```python
from build123d import *

# Parameters (mm, degrees)
SKETCH1_W               = 5.7
SKETCH1_H               = 3.4
SKETCH1_W_2             = 36.24
SKETCH1_H_2             = 45
BOSS_EXTRUDE1_DEPTH     = 3
CUT_EXTRUDE1_DEPTH      = 61
CUT_EXTRUDE1_DEPTH_BACK = 19
SKETCH3_W               = 24.5
SKETCH3_H               = 2.46523088
BOSS_EXTRUDE2_DEPTH     = 2


with BuildPart() as part:
    # Sketch1 → Boss-Extrude1 (new body)
    with BuildSketch(Plane(origin=(0, 0, 0), x_dir=(1, 0, 0), z_dir=(0, 1, 0))):
        Polygon((85, 0), (0, 0), (0, -23), (8.59, -23), (8.59, -32), (0, -32), (0, -55), (85, -55), align=None)
        Polygon((9.59, -33.35), (9.59, -32.35), (9.59, -22.65), (9.59, -21.65), (13.68, -21.65), (13.68, -33.35), align=None, mode=Mode.SUBTRACT)
        with Locations((73.3, -27.5)):
            Rectangle(SKETCH1_W, SKETCH1_H, mode=Mode.SUBTRACT)
        with Locations((45.38, -27.5)):
            Rectangle(SKETCH1_W_2, SKETCH1_H_2, mode=Mode.SUBTRACT)
    extrude(amount=BOSS_EXTRUDE1_DEPTH)

    # Sketch3 → Cut-Extrude1 (cut, two sides: drawn at the far end of the back side and taken through both)
    with BuildSketch(Plane.ZY.offset(-63.5).offset(-CUT_EXTRUDE1_DEPTH_BACK)):
        with Locations((27.5, 1.23261544)):
            Rectangle(SKETCH3_W, SKETCH3_H)
    extrude(amount=CUT_EXTRUDE1_DEPTH + CUT_EXTRUDE1_DEPTH_BACK, mode=Mode.SUBTRACT)

    # Sketch4 → Boss-Extrude2 (add)
    with BuildSketch(Plane.XZ):
        Polygon((0, 32), (2.5, 32), (2.5, 39.75), (2.5, 52.5), (82.5, 52.5), (82.5, 39.75), (82.5, 15.25), (82.5, 2.5), (2.5, 2.5), (2.5, 15.25), (2.5, 23), (0, 23), (0, 0), (85, 0), (85, 55), (0, 55), align=None)
    extrude(amount=BOSS_EXTRUDE2_DEPTH)


solid = part.part
```
Geometry: final body of the model. Coordinates: model frame, mm. A direction names the side the tool comes from. Give positions to 0.01 mm unless a question says otherwise; leave off trailing zeros. Write each loop counter-clockwise with the first axis right and the second up, starting at its lowest first coordinate (ties: lowest second). Pieces come first, ordered by that corner, then holes.
1. Section query C-C, the plane y = 0.8. Return loops of the section in (x, z), then the cut area to 3 significant figures.
2. Draft query along X for faces 1 (the flat face through (0, 1, 44)), 2 (the flat face through (43, 1, 55)), 3 (the flat face through (42, -1, 52.5)). Return one class per face: released by +X, released by -X, zero draft, split by the parting line, or undercut.
3. Section query D-D, the plane x = 57. Return loops of the section in (y, z).
4. Section query B-B, the plane x = 19. Return loops of the section in (y, z).
5. Reachability of faces 4 (the flat face through (27.26, 2.8, 27.8)), 5 (the flat face through (2, 1, 32)), 6 (the flat face through (42, 1, 0)), 7 (the flat face through (0, 1, 12)), 8 (the flat face through (43, -1, 2.5)) from +Z, -Z, +X, -X, +Y, -Y: full face, straight path, thin tool, end or side. Return the list, or none.
6. Line query: probe 1 along Z at (x, y) = (72.5, -1.3); probe 2 along X at (y, z) = (2.45, 7); probe 3 along Z at (x, y) = (15.5, 2.25). Output: solid intervals per line, ascending.
7. Pin query (flat end, axial travel): P1, Ø1, axis at y = 0, z = 24.5, coming from the -X side; P2, Ø0.6, axis at y = 3, z = 26.5, coming from the -X side; P3, Ø6.5, axis at x = 27, z = 8.5, coming from the -Y side. Return the tip coordinate at first contact, or that it passes through.
8. Section query A-A, the plane z = 42. Return loops of the section in (x, y), then the cut area to 3 significant figures.
Computed:
1. outline: (0, 0) - (85, 0) - (85, 55) - (0, 55) - (0, 32) - (2.5, 32) - (2.5, 39.75) - (27.26, 39.75) - (27.26, 50) - (63.5, 50) - (63.5, 39.75) - (82.5, 39.75) - (82.5, 15.25) - (63.5, 15.25) - (63.5, 5) - (27.26, 5) - (27.26, 15.25) - (2.5, 15.25) - (2.5, 23) - (0, 23) - close
1. area: 1,950 mm2
2. face 1: released by -X
2. face 2: zero draft
2. face 3: undercut
3. outline: (-2, 0) - (3, 0) - (3, 5) - (0, 5) - (0, 2.5) - (-2, 2.5) - close; (-2, 52.5) - (0, 52.5) - (0, 50) - (3, 50) - (3, 55) - (-2, 55) - close
4. outline: (-2, 0) - (3, 0) - (3, 55) - (-2, 55) - (-2, 52.5) - (0, 52.5) - (0, 39.75) - (2.47, 39.75) - (2.47, 15.25) - (0, 15.25) - (0, 2.5) - (-2, 2.5) - close
5. face 4: +Y, -Y
5. face 5: -X, +Y, -Y
5. face 6: -Z, +X, -X, +Y, -Y
5. face 7: +Z, -Z, -X, +Y, -Y
5. face 8: -Y
6. probe 1: z = 0 to 2.5, 52.5 to 55
6. probe 2: x = 0 to 27.26, 63.5 to 85
6. probe 3: z = 0 to 15.25, 39.75 to 55
7. P1: stops at x = 82.5
7. P2: stops at x = 8.59
7. P3: stops at y = 0
8. outline: (0, -2) - (2.5, -2) - (2.5, 0) - (27.26, 0) - (27.26, 3) - (0, 3) - close; (63.5, 0) - (82.5, 0) - (82.5, -2) - (85, -2) - (85, 3) - (63.5, 3) - close
8. area: 156 mm2
